The model under review builds one solid part; all positions refer to its coordinate system, in mm. Face numbers are marked on the shaded views. A direction names the side the tool comes from. Coordinates: 2 decimals unless noted, no trailing zeros. Write each loop counter-clockwise with the first axis right and the second up, starting at its lowest first coordinate (ties: lowest second). Pieces come first, ordered by that corner, then holes. Notation, with made-up numbers: (-17, -30) - (25, -30) arc R13 cw to (25, -7) - close; hole circle Ø9 at (58, 0.25). An arc over 180 degrees is marked (long way). Put each result on its own line as item: value. Start each with the question number.
Item 1: To check wall thickness, follow L1, parallel to X at y = 0.6, z = -10; L2, parallel to X at y = 1.65, z = -10. State the ranges of each line that lie inside material, in increasing order. Write a range as [from, to].
Item 2: For pin 1 (1.3 mm diameter, centred on x = -10, z = -9.5, fed in from +Y); pin 2 (3.5 mm diameter, centred on x = 10, z = 10, fed in from +Y), all flat-tipped, find the tip position at first contact; note any pin that passes through.
Item 3: Mouldability with a two-part tool opening along X and no side actions: class the marked faces 1 and 2 as pulls with the +X half, pulls with the -X half, needs draft (parallel to the pull), parting line crosses it, or undercut.
Item 4: Consider section B-B on x = -10. Give the boundary of the cut face in (y, z).
Item 5: Consider section A-A on z = -10. Give the boundary of the cut face in (x, y).
Item 6: Consider section D-D on x = 1.75. Give the boundary of the cut face in (y, z).
Item 7: Machinability: for the marked faces 3 and 4, which of the approach directions +Z, -Z, +X, -X, +Y, -Y give a long, thin tool a straight path to every point of the face, cutting with its end or side? Answer none if there is none.
Item 8: Consider section C-C on y = 1.8. Give the boundary of the cut face in (x, z).
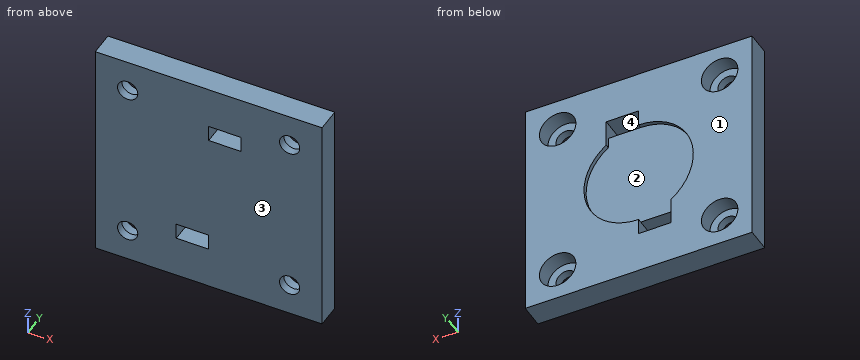
Autodesk Fusion 360 part; units mm, degrees
sketch "Sketch1" plane through (0, 0, 0) normal (0, 1, 0) x (1, 0, 0)
  line L0 (-14, 14) -> (14, 14)
  line L1 (14, 14) -> (14, -14)
  line L2 (14, -14) -> (-14, -14)
  line L3 (-14, -14) -> (-14, 14)
  line L4 (-14, 14) -> (14, -14) construction
  circle A0 centre (0, 0) radius 6.75
  line L5 (-4, 8.75) -> (0, 8.75)
  line L6 (0, 8.75) -> (0, 6.75)
  line L7 (0, 6.75) -> (-4, 6.75)
  line L8 (-4, 6.75) -> (-4, 8.75)
  line L9 (0, 0) -> (0, 6.75)
  line L10 (0, 0) -> (0, -6.75)
  line L11 (0, -6.75) -> (4, -6.75)
  line L12 (4, -6.75) -> (4, -8.75)
  line L13 (4, -8.75) -> (0, -8.75)
  line L14 (0, -8.75) -> (0, -6.75)
  line L15 (10, -10) -> (-10, -10) construction
  line L16 (-10, -10) -> (-10, 10) construction
  line L17 (-10, 10) -> (10, 10) construction
  line L18 (10, 10) -> (10, -10) construction
  circle A1 centre (-10, 10) radius 1.25
  circle A2 centre (10, 10) radius 1.25
  circle A3 centre (-10, -10) radius 1.25
  circle A4 centre (10, -10) radius 1.25
  line L19 (4, -6.75) -> (4, -5.4371)
  line L20 (-4, 6.75) -> (-4, 5.4371)
  circle A5 centre (-10, -10) radius 2.25
  circle A6 centre (-10, 10) radius 2.25
  circle A7 centre (10, 10) radius 2.25
  circle A8 centre (10, -10) radius 2.25
  dimension "d1" = 28
  dimension "d2" = 28
  dimension "d3" = 13.5
  dimension "d4" = 4
  dimension "d5" = 2
  dimension "d8" = 4
  dimension "d9" = 2
  dimension "d10" = 4
  dimension "d11" = 2.5
  dimension "d12" = 2.5
  dimension "d13" = 2.5
  dimension "d14" = 2.5
  dimension "d20" = 4.5
  dimension "d21" = 4.5
  dimension "d22" = 4.5
  dimension "d23" = 4.5
extrude "Extrude1" add sketch "Sketch1" along normal blind 3 contours L0 L1 L2 L3 | A0 L9 L10 | A0 L9 L10 | A0 L7 L20 | A0 L11 L19 | A5 | A6 | A7 | A8
extrude "Extrude2" cut sketch "Sketch1" against normal blind 0.5 from surface at 3 contours A0 L9 L10 | A0 L9 L10 | A0 L7 L20 | A0 L11 L19
extrude "Extrude3" cut sketch "Sketch1" against normal blind 2 from surface at 3 contours A2 | A5 | A6 | A7 | A8
equation "d1 = d2"
Report:
1. L1: [-14, -11.25], [-8.75, 8.75], [11.25, 14]
1. L2: [-14, -12.25], [-7.75, 7.75], [12.25, 14]
2. pin 1: through
2. pin 2: y = 1
3. face 1: needs draft
3. face 2: undercut
4. outline: (0, -14) - (3, -14) - (3, -12.25) - (1, -12.25) - (1, -11.25) - (0, -11.25) - close; (0, -8.75) - (1, -8.75) - (1, -7.75) - (3, -7.75) - (3, 7.75) - (1, 7.75) - (1, 8.75) - (0, 8.75) - close; (0, 11.25) - (1, 11.25) - (1, 12.25) - (3, 12.25) - (3, 14) - (0, 14) - close
5. outline: (-14, 0) - (-11.25, 0) - (-11.25, 1) - (-12.25, 1) - (-12.25, 3) - (-14, 3) - close; (-8.75, 0) - (8.75, 0) - (8.75, 1) - (7.75, 1) - (7.75, 3) - (-7.75, 3) - (-7.75, 1) - (-8.75, 1) - close; (11.25, 0) - (14, 0) - (14, 3) - (12.25, 3) - (12.25, 1) - (11.25, 1) - close
6. outline: (0, -14) - (3, -14) - (3, -6.52) - (2.5, -6.52) - (2.5, 6.75) - (0, 6.75) - close; (0, 8.75) - (3, 8.75) - (3, 14) - (0, 14) - close
7. face 3: +Z, -Z, +X, -X, -Y
7. face 4: +Y, -Y
8. outline: (-14, -14) - (14, -14) - (14, 14) - (-14, 14) - close; hole circle Ø4.5 at (-10, -10); hole circle Ø4.5 at (-10, 10); hole (-4, -8.75) - (0, -8.75) - (0, -6.75) - (-4, -6.75) - close; hole (0, 6.75) - (4, 6.75) - (4, 8.75) - (0, 8.75) - close; hole circle Ø4.5 at (10, -10); hole circle Ø4.5 at (10, 10)
